Here's how the part is built. I have some questions about the finished solid (model axes, mm). A direction names the side the tool comes from. Coordinates: 2 decimals unless noted, no trailing zeros. Write each loop counter-clockwise with the first axis right and the second up, starting at its lowest first coordinate (ties: lowest second). Pieces come first, ordered by that corner, then holes.
Item 1: If we section it at B-B (x = 69.5): Please give me the cut outline in (y, z).
Item 2: For faces 1 (the face through (107.07, 32.56, 33.54)), 2 (the face through (76, 30, 65)), 3 (the face through (37.17, 25.24, -0.99)), which set-ups out of +Z, -Z, +X, -X, +Y, -Y let a thin tool reach every point of the face, with its end or its side?
Item 3: I'm going to push flat-ended pins straight in: pin 1 Ø10 at (x, z) = (12, 19) entering from +Y; pin 2 Ø21 at (x, y) = (56.5, 25.5) entering from +Z; pin 3 Ø4 at (x, y) = (69, 23) entering from -Z; pin 4 Ø8 at (x, y) = (35, 35) entering from +Z. Where does each tip first touch, or does it pass through?
Item 4: If I drill on line 1 (Y direction, x = 105.75, z = 33); line 2 (X direction, y = 35, z = 12.5); line 3 (Z direction, x = 51.5, y = 8), over which ranges is the centre line in solid material (lowest first)?
Item 5: If we section it at A-A (z = 33): Please give me the cut outline in (x, y), then the cut area to 3 significant figures.
Item 6: We'd pull the mould along Z, two halves only. Please class faces 4 (the face through (33, 33, -2)), 5 (the face through (82.19, 43.79, 5.08)), 6 (the face through (102, 35, 33)): +Z half, -Z half, draft (parallel to the pull), parting line (faces both ways), or undercut.
Item 7: If we section it at C-C (x = 17.5): Please give me the cut outline in (y, z).
from build123d import *

# Parameters (mm, degrees)
SKETCH_1_W          = 76
SKETCH_1_H          = 70
EXTRUDE_1_DEPTH     = 66
CUT_EXTRUDE_1_DEPTH = 123.605056992
SKETCH_3_R          = 2.5
CUT_EXTRUDE_2_DEPTH = 123.605056992
SKETCH_4_R          = 29
EXTRUDE_2_DEPTH     = 6
FILLET_1_R          = 3
SKETCH_5_R          = 33.5
EXTRUDE_3_DEPTH     = 30
CHAMFER_2_SIZE      = 4
CHAMFER_2_SIZE2     = 4.442450059
SKETCH_6_R          = 2.5
CUT_EXTRUDE_3_DEPTH = 10
EXTRUDE_START       = 2
SKETCH_7_R          = 10
SKETCH_7_R_2        = 2.5
EXTRUDE_4_DEPTH     = 2
SKETCH_8_R          = 10
SKETCH_8_R_2        = 2.5
EXTRUDE_5_DEPTH     = 2


with BuildPart() as part:
    # ｽｹｯﾁ1 → 押し出し1 (new body)
    with BuildSketch(Plane.XY):
        with Locations((38, 35)):
            Rectangle(SKETCH_1_W, SKETCH_1_H)
    extrude(amount=EXTRUDE_1_DEPTH)

    # ｽｹｯﾁ2 → ｶｯﾄ - 押し出し1 (cut, through all)
    with BuildSketch(Plane.XY.offset(66)):
        with BuildLine():
            ThreePointArc((0, 35), (10.251262658, 59.748737342), (35, 70))
            Line((35, 70), (0, 70))
            Line((0, 70), (0, 35))
        make_face()
        with BuildLine():
            Line((0, 0), (35, 0))
            ThreePointArc((35, 0), (10.251262658, 10.251262658), (0, 35))
            Line((0, 35), (0, 0))
        make_face()
    extrude(amount=-CUT_EXTRUDE_1_DEPTH, mode=Mode.SUBTRACT)

    # ｽｹｯﾁ3 → ｶｯﾄ - 押し出し2 (cut, through all)
    with BuildSketch(Plane.XY.offset(66)):
        with Locations((35, 35)):
            Circle(SKETCH_3_R)
    extrude(amount=-CUT_EXTRUDE_2_DEPTH, mode=Mode.SUBTRACT)

    # ｽｹｯﾁ4 → 押し出し2 (add)
    with BuildSketch(Plane(origin=(76, 0, 0), x_dir=(0, 0, -1), z_dir=(1, 0, 0))):
        with Locations(Location((-33, 35, 0), (0, 0, 180))):
            Circle(SKETCH_4_R)
    extrude(amount=EXTRUDE_2_DEPTH)

    # ﾌｨﾚｯﾄ1
    fillet_1_edges = [part.edges().sort_by_distance(p)[0] for p in [
        (76, 35, 4),
    ]]
    fillet(fillet_1_edges, radius=FILLET_1_R)

    # ｽｹｯﾁ5 → 押し出し3 (add)
    with BuildSketch(Plane(origin=(82, 0, 0), x_dir=(0, 0, -1), z_dir=(1, 0, 0))):
        with Locations((-33, 35)):
            Circle(SKETCH_5_R)
    extrude(amount=EXTRUDE_3_DEPTH)

    # 面取り2
    chamfer_2_edges = [part.edges().sort_by_distance(p)[0] for p in [
        (82, 35, 66.5),
    ]]
    chamfer_2_side = [part.faces().sort_by_distance(p)[0] for p in [
        (97, 35, 66.5),
    ]]
    chamfer(chamfer_2_edges, length=CHAMFER_2_SIZE, length2=CHAMFER_2_SIZE2, reference=chamfer_2_side[0])

    # ｽｹｯﾁ6 → ｶｯﾄ - 押し出し3 (cut)
    with BuildSketch(Plane(origin=(112, 0, 0), x_dir=(0, 0, -1), z_dir=(1, 0, 0))):
        with Locations((-33, 35)):
            Circle(SKETCH_6_R)
    extrude(amount=-CUT_EXTRUDE_3_DEPTH, mode=Mode.SUBTRACT)

    # ｽｹｯﾁ7 → 押し出し4 (add)
    with BuildSketch(Plane.XY.offset(66).offset(EXTRUDE_START)):
        with Locations(Location((35, 35, 0), (0, 0, 180))):
            Circle(SKETCH_7_R)
        with Locations((35, 35)):
            Circle(SKETCH_7_R_2, mode=Mode.SUBTRACT)
    extrude(amount=-EXTRUDE_4_DEPTH)

    # ｽｹｯﾁ8 → 押し出し5 (add)
    with BuildSketch(Plane(origin=(0, 0, 0), x_dir=(-1, 0, 0), z_dir=(0, 0, -1))):
        with Locations((-35, 35)):
            Circle(SKETCH_8_R)
        with Locations(Location((-35, 35, 0), (0, 0, 180))):
            Circle(SKETCH_8_R_2, mode=Mode.SUBTRACT)
    extrude(amount=EXTRUDE_5_DEPTH)


solid = part.part
Answer list:
1. outline: (0, 0) - (70, 0) - (70, 66) - (0, 66) - close
2. face 1: +X
2. face 2: none
2. face 3: -Z
3. pin 1: stops at y = 65.02
3. pin 2: stops at z = 66
3. pin 3: stops at z = 0
3. pin 4: stops at z = 68
4. line 1: y = 1.5 to 32.5, 37.5 to 68.5
4. line 2: x = 0 to 32.5, 37.5 to 112
4. line 3: z = 0 to 66
5. outline: (35, 0) - (76, 0) - (76, 3) arc R3 cw to (79, 6) - (82, 6) - (82, 5.94) - (86, 1.5) - (112, 1.5) - (112, 32.5) - (102, 32.5) - (102, 37.5) - (112, 37.5) - (112, 68.5) - (86, 68.5) - (82, 64.06) - (82, 64) - (79, 64) arc R3 cw to (76, 67) - (76, 70) - (35, 70) arc R35 ccw to start; hole circle Ø5 at (35, 35)
5. area: 7,070 mm2
6. face 4: -Z half
6. face 5: parting line
6. face 6: undercut
7. outline: (4.69, 0) - (65.31, 0) - (65.31, 66) - (4.69, 66) - close
